Could you check a few things on this model? Use its own coordinates, in mm. A direction names the side the tool comes from. Coordinates: 2 decimals unless noted, no trailing zeros. Write each loop counter-clockwise with the first axis right and the second up, starting at its lowest first coordinate (ties: lowest second). Pieces come first, ordered by that corner, then holes.
```python
from build123d import *

# Parameters (mm, degrees)
ESQUISSE1_W             = 14
ESQUISSE1_H             = 10
BOSS_EXTRU_1_DEPTH      = 10
ESQUISSE4_R             = 4
BOSS_EXTRU_2_DEPTH      = 5
ESQUISSE5_R             = 2.5
ENL_V_MAT_EXTRU_2_DEPTH = 5
CONG_3_R                = 1
CONG_4_R                = 1
ESQUISSE6_W             = 10
ESQUISSE6_H             = 10
ENL_V_MAT_EXTRU_3_DEPTH = 5


with BuildPart() as part:
    # Esquisse1 → Boss.-Extru.1 (new body)
    with BuildSketch(Plane.XY):
        with Locations((7, 5)):
            Rectangle(ESQUISSE1_W, ESQUISSE1_H)
    extrude(amount=BOSS_EXTRU_1_DEPTH)

    # Esquisse4 → Boss.-Extru.2 (add)
    with BuildSketch(Plane(origin=(0, 0, 0), x_dir=(-1, 0, 0), z_dir=(0, 0, -1))):
        with Locations((-7, 5)):
            Circle(ESQUISSE4_R)
    extrude(amount=BOSS_EXTRU_2_DEPTH)

    # Esquisse5 → Enlèv. mat.-Extru.2 (cut)
    with BuildSketch(Plane(origin=(0, 0, -5), x_dir=(-1, 0, 0), z_dir=(0, 0, -1))):
        with Locations((-7, 5)):
            Circle(ESQUISSE5_R)
    extrude(amount=-ENL_V_MAT_EXTRU_2_DEPTH, mode=Mode.SUBTRACT)

    # Congé3
    cong_3_edges = [part.edges().sort_by_distance(p)[0] for p in [
        (11, 5, 0),
    ]]
    fillet(cong_3_edges, radius=CONG_3_R - 0.0001)  # a hair under: the kernel refuses the full size

    # Congé4
    cong_4_edges = [part.edges().sort_by_distance(p)[0] for p in [
        (14, 5, 0),
        (0, 5, 0),
    ]]
    fillet(cong_4_edges, radius=CONG_4_R)

    # Esquisse6 → Enlèv. mat.-Extru.3 (cut)
    with BuildSketch(Plane.XY.offset(10)):
        with Locations((7, 5)):
            Rectangle(ESQUISSE6_W, ESQUISSE6_H)
    extrude(amount=-ENL_V_MAT_EXTRU_3_DEPTH, mode=Mode.SUBTRACT)


solid = part.part
```
Item 1: Will this pin go through, and if not, where does the flat tip stop? pin 1 Ø5 at (x, y) = (10.5, 8.5) entering from -Z.
Item 2: I want a section at A-A, the plane z = 9.25. List the corners of the cut face in (x, y) for me, then the cut area to 3 significant figures.
Item 3: I want a section at B-B, the plane y = 5. List the corners of the cut face in (x, z) for me.
Item 4: Which directions (+Z, -Z, +X, -X, +Y, -Y) give clear straight access to the entire face, cutting with the end or side of a thin tool? Please do faces 4 (the cylindrical face through (0.301, 5.07, 0.285)), 5 (the flat face through (12, 5, 8)), 6 (the flat face through (7, 5, 0)).
Item 5: If we mould it in two halves opening along Y, with no side actions, what happens to faces 1 (the cylindrical face through (4.615, 5.751, -2.535)), 2 (the flat face through (2, 5, 8)), 3 (the flat face through (7, 10, 4))? For each: released by +Y, released by -Y, zero draft, split by the parting line, or undercut.
Item 6: If I drill on line 1 along Y through (x, z) = (7, -2.55); line 2 along X through (y, z) = (8.25, 9.25); line 3 along Z through (x, y) = (11.5, 2), over which ranges is the centre line in solid material (lowest first)?
Item 7: I want a section at D-D, the plane z = -0.75. List the corners of the cut face in (x, y) for me.
Taken from the geometry:
1. pin 1: stops at z = -5
2. outline: (0, 0) - (2, 0) - (2, 10) - (0, 10) - close; (12, 0) - (14, 0) - (14, 10) - (12, 10) - close
2. area: 40.0 mm2
3. outline: (0, 1) arc R1 ccw to (1, 0) - (2, 0) arc R1 cw to (3, -1) - (3, -5) - (4.5, -5) - (4.5, 0) - (9.5, 0) - (9.5, -5) - (11, -5) - (11, -1) arc R1 cw to (12, 0) - (13, 0) arc R1 ccw to (14, 1) - (14, 10) - (12, 10) - (12, 5) - (2, 5) - (2, 10) - (0, 10) - close
4. face 4: -Z, -X, +Y, -Y
4. face 5: +Z, +Y, -Y
4. face 6: -Z
5. face 1: undercut
5. face 2: zero draft
5. face 3: released by +Y
6. line 1: y = 1 to 2.5, 7.5 to 9
6. line 2: x = 0 to 2, 12 to 14
6. line 3: z = 0 to 5
7. outline: circle Ø8.06 at (7, 5); hole circle Ø5 at (7, 5)
